Autodesk Inventor part; units mm, degrees
ref_plane "YZ Plane" through (0, 0, 0) normal (1, 0, 0) x (0, 1, 0)
ref_plane "XZ Plane" through (0, 0, 0) normal (0, 1, 0) x (-1, 0, 0)
ref_plane "XY Plane" through (0, 0, 0) normal (0, 0, 1) x (1, 0, 0)
sketch "Szkic1" plane through (0, 0, 0) normal (0, 1, 0) x (-1, 0, 0)
  line L0 (0, 0) -> (-49.134, 0)
  line L1 (-49.134, 1) -> (0, 1)
  line L2 (0, 1) -> (0, 0)
  circle A0 centre (-50, 0.5) radius 1
  circle A1 centre (-50, 0.5) radius 0.5
  dimension "d2" = 2
  dimension "d3" = 1
  dimension "d4" = 49.134
  dimension "d9" = 1
extrude "Wyciągnięcie proste1" add sketch "Szkic1" along normal blind 50 contours L0 A0 L1 L2
extrude "Wyciągnięcie proste3" add sketch "Szkic1" along normal blind 25 contours A0
properties part number "zawias"
CAD build for the part. Positions are in the model's coordinates, mm. A direction names the side the tool comes from. Give positions to 0.01 mm unless a question says otherwise; leave off trailing zeros. Loops run counter-clockwise (first coordinate to the right, second up) from the corner with the lowest first, then second, coordinate; pieces in that order, holes last. Notation, with made-up numbers: (76.5, 35.5) - (82.5, 35.5) arc R21 ccw to (82.5, 41.5) - close; hole circle Ø8 at (84, -24). An arc over 180 degrees is marked (long way). Put each result on its own line as item: value.
Q1. Flat gauge pins, fed straight in: pin 1 (14.5 mm diameter, centred on x = 33, y = 23.5, fed in from +Z); pin 2 (1 mm diameter, centred on x = 50, z = 1, fed in from +Y); pin 3 (8 mm diameter, centred on x = 20.5, y = 24, fed in from -Z). Where does each tip first touch, or does it go through?
Filled in:
pin 1: stops at z = 1
pin 2: stops at y = 25
pin 3: stops at z = 0
Q2. Slice it at D-D (y = 36). Give the cut face in (x, z), plus the area to 3 significant figures.
Filled in:
outline: (0, 0) - (49.13, 0) arc R1 cw to (49.13, 1) - (0, 1) - close
area: 49.0 mm²
Q3. Slice it at A-A (z = 0.5). Give the cut face in (x, y).
Filled in:
outline: (0, 0) - (49.5, 0) - (49.5, 25) - (49, 25) - (49, 50) - (0, 50) - close; (50.5, 0) - (51, 0) - (51, 25) - (50.5, 25) - close
Q4. Slice it at C-C (x = 12). Give the cut face in (y, z).
Filled in:
outline: (0, 0) - (50, 0) - (50, 1) - (0, 1) - close
Q5. Slice it at B-B (y = 24). Give the cut face in (x, z), plus the area to 3 significant figures.
Filled in:
outline: (0, 0) - (49.13, 0) arc R1 ccw (long way) to (49.13, 1) - (0, 1) - close; hole circle Ø1 at (50, 0.5)
area: 51.4 mm²
Q6. Probe line 1 along Z through (x, y) = (50, 5); line 2 along X through (y, z) = (4, 0.45); line 3 along Z through (x, y) = (14, 44.5). List the from-to ranges inside material, lowest first.
Filled in:
line 1: z = -0.5 to 0, 1 to 1.5
line 2: x = 0 to 49.5, 50.5 to 51
line 3: z = 0 to 1
Q7. Tool access for faces 1 (the face through (25, 25, 1)), 2 (the face through (24, 25, 0)), 3 (the face through (51, 12.3, 0.5)): list every direction of +Z, -Z, +X, -X, +Y, -Y with a clear straight run to the whole face (end or side of a thin tool).
Filled in:
face 1: +Z, -X, +Y, -Y
face 2: -Z, -X, +Y, -Y
face 3: +Y, -Y
